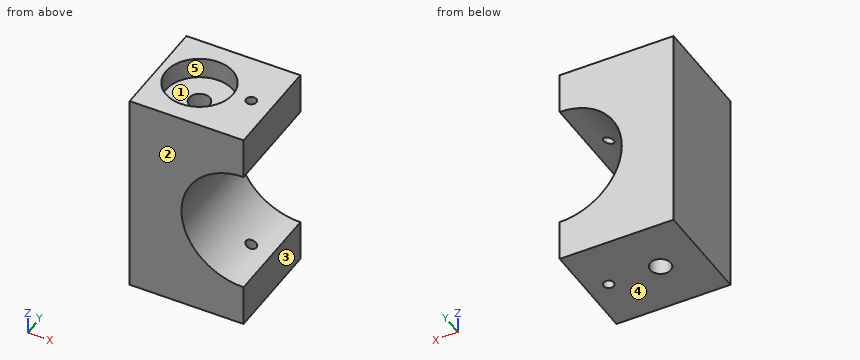
Autodesk Inventor part; units mm, degrees
ref_plane "YZ Plane" through (0, 0, 0) normal (1, 0, 0) x (0, 1, 0)
ref_plane "XZ Plane" through (0, 0, 0) normal (0, 1, 0) x (-1, 0, 0)
ref_plane "XY Plane" through (0, 0, 0) normal (0, 0, 1) x (1, 0, 0)
sketch "Sketch1" plane through (0, 0, 0) normal (0, 1, 0) x (-1, 0, 0)
  line L0 (0, -50) -> (55, -50)
  line L1 (55, -50) -> (55, 50)
  line L2 (55, 50) -> (0, 50)
  arc A0 (0, -30) -> (0, 30) centre (0, 0) ccw
  line L3 (0, 50) -> (0, 30)
  line L4 (0, -30) -> (0, -50)
  point P0 (55, 0)
  dimension "d0" = 100
  dimension "d1" = 55
  dimension "d3" = 60
extrude "Extrusion1" add sketch "Sketch1" along normal blind 50
sketch "Sketch2" plane through (-55, 0, 50) normal (0, 0, 1) x (1, 0, 0)
  line L0 (55, 0) -> (55, 50) construction
  line L1 (55, 50) -> (0, 50) construction
  line L2 (55, 0) -> (0, 0) construction
  line L3 (0, 0) -> (0, 50)
  point P0 (20, 25)
  point P1 (0, 25)
  dimension "d14" = 20
hole "Hole1" at (-35, 25, 50) direction (0, 0, -1) diameter 10 end through all counterbore diameter 32.4 counterbore depth 10
sketch "Sketch4" plane through (0, 0, -50) normal (0, 0, -1) x (-1, 0, 0)
  line L0 (55, 0) -> (55, 50)
  line L1 (0, 0) -> (0, 50)
  point P0 (10, 25)
  point P1 (55, 25)
  dimension "d15" = 10
hole "Hole2" at (-10, 25, -50) direction (0, 0, 1) diameter 5 end through all
properties part number "acople_tubo"
Could you check a few things on this model? Use its own coordinates, in mm. Face numbers are marked on the shaded views. A direction names the side the tool comes from. Round coordinates to 2 decimals unless told otherwise and drop trailing zeros. Order: outer loops, then holes, each group sorted by start corner. A loop starts at its lowest first (then second) coordinate and runs counter-clockwise, first axis right, second up.
(1) Imagine slicing it at A-A (x = -35). Write out the boundary of the cut face in (y, z).
Response values:
outline: (0, -50) - (20, -50) - (20, 40) - (8.8, 40) - (8.8, 50) - (0, 50) - close; (30, -50) - (50, -50) - (50, 50) - (41.2, 50) - (41.2, 40) - (30, 40) - close
(2) Imagine slicing it at B-B (z = 0). Write out the boundary of the cut face in (x, y), plus the area to 3 significant figures.
Response values:
outline: (-55, 0) - (-30, 0) - (-30, 50) - (-55, 50) - close; hole circle Ø10 at (-35, 25)
area: 1,170 mm2
(3) I'm going to push a flat-ended pin straight in: pin 1 (3 mm diameter, centred on y = 14.5, z = -3, fed in from +X). Where does the tip first touch, or does it pass through?
Response values:
pin 1: stops at x = -29.66
(4) Imagine slicing it at D-D (y = 47.5). Write out the boundary of the cut face in (x, z).
Response values:
outline: (-55, -50) - (0, -50) - (0, -30) arc R30 cw to (0, 30) - (0, 50) - (-55, 50) - close
(5) Which directions (+Z, -Z, +X, -X, +Y, -Y) give clear straight access to the entire face, cutting with the end or side of a thin tool? Please do the marked faces 1 and 2.
Response values:
face 1: +Z
face 2: +Z, -Z, +X, -X, -Y
(6) If we mould it in two halves opening along X, with no side actions, what happens to the marked faces 3, 4 and 5? For each: released by +X, released by -X, zero draft, split by the parting line, or undercut.
Response values:
face 3: released by +X
face 4: zero draft
face 5: undercut
(7) Imagine slicing it at C-C (x = -10). Write out the boundary of the cut face in (y, z), plus the area to 3 significant figures.
Response values:
outline: (0, -50) - (22.5, -50) - (22.5, -28.28) - (0, -28.28) - close; (0, 28.28) - (22.5, 28.28) - (22.5, 50) - (0, 50) - close; (27.5, -50) - (50, -50) - (50, -28.28) - (27.5, -28.28) - close; (27.5, 28.28) - (50, 28.28) - (50, 50) - (27.5, 50) - close
area: 1,950 mm2
(8) Please list where these lines run through material, in increasing order: line 1 along X through (y, z) = (25, 38); line 2 along X through (y, z) = (25, 43); line 3 along Y through (x, z) = (-35, -29).
Response values:
line 1: x = -55 to -40, -30 to -12.5, -7.5 to 0
line 2: x = -55 to -51.2, -18.8 to -12.5, -7.5 to 0
line 3: y = 0 to 20, 30 to 50
